Study the drawing (mm; zero at the part's minimum x, y, z) and answer. A direction names the side the tool comes from. Coordinates: 2 decimals unless noted, no trailing zeros. Loops run counter-clockwise (first coordinate to the right, second up) from the corner with the lowest first, then second, coordinate; pieces in that order, holes last.
Q1. Section A-A (z = 9) is taken. Give the vertices of the cut face in (x, y) (3 decimals), then the cut area to 3 significant figures.
Q2. Which of the six approach directions +Z, -Z, +X, -X, +Y, -Y give full straight-line access (tool end or side, diameter ignored) to the marked faces 1 and 2?
Q3. Flat-ended cylindrical pins translate along their axes: P1, Ø5, axis at y = 16, z = 31.5, coming from the -X side (3 decimals); P2, Ø10, axis at x = 25, y = 19.5, coming from the -Z side; P3, Ø4, axis at x = 13, z = 16, coming from the -Y side (3 decimals). Find the tip coordinate at first contact, or state that the pin passes through.
Q4. Straight lines are drawn through the part: line 1 (Y direction, x = 11.5, z = 26) (3 decimals); line 2 (Y direction, x = 36.5, z = 33.5). For each, find the intervals that lie inside material, in ascending order.
Q5. Section B-B (x = 14) is taken. Give the vertices of the cut face in (y, z) (3 decimals), then the cut area to 3 significant figures.
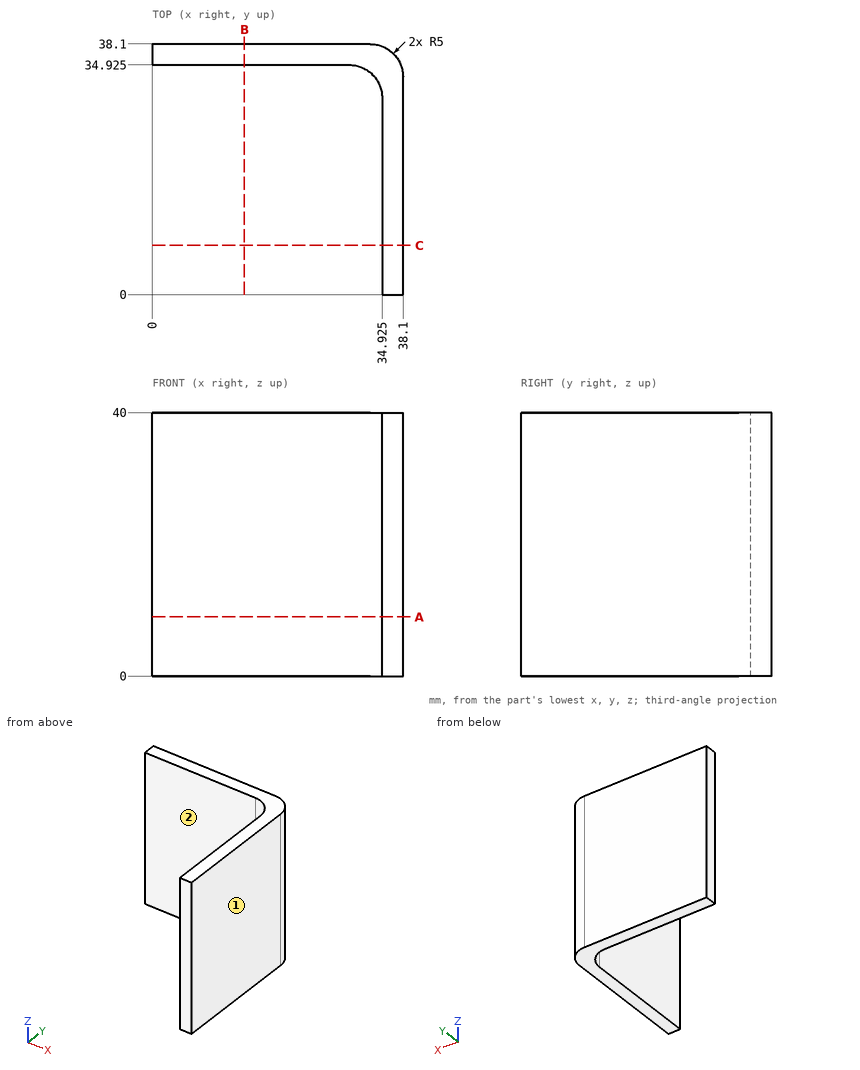
Numbers:
1. outline: (0, 34.925) - (29.925, 34.925) arc R5 cw to (34.925, 29.925) - (34.925, 0) - (38.1, 0) - (38.1, 33.1) arc R5 ccw to (33.1, 38.1) - (0, 38.1) - close
1. area: 232 mm2
2. face 1: +Z, -Z, +X, +Y, -Y
2. face 2: +Z, -Z, -X, -Y
3. P1: stops at x = 34.925
3. P2: passes through
3. P3: stops at y = 34.925
4. line 1: y = 34.925 to 38.1
4. line 2: y = 0 to 36.77
5. outline: (34.925, 0) - (38.1, 0) - (38.1, 40) - (34.925, 40) - close
5. area: 127 mm2
